Read the model definition and answer for the solid it produces. Units are mm, in the model's axes. Face numbers are marked on the shaded views. A direction names the side the tool comes from. Coordinates: 2 decimals unless noted, no trailing zeros. Write each loop counter-clockwise with the first axis right and the second up, starting at its lowest first coordinate (ties: lowest second). Pieces come first, ordered by that corner, then holes.
1) The part is cut by section D-D (y = 47.5). Determine the outline of the cut face in (x, z), then the cut area to 3 significant figures.
2) The part is cut by section C-C (y = 54). Determine the outline of the cut face in (x, z), then the cut area to 3 significant figures.
3) The part is cut by section B-B (x = 0). Determine the outline of the cut face in (y, z), then the cut area to 3 significant figures.
4) Each of these flat-tipped pins is pushed along its axis until it touches: pin 1 Ø4 at (y, z) = (27, -20) entering from +X; pin 2 Ø6 at (x, z) = (10, 12.5) entering from -Y; pin 3 Ø12 at (y, z) = (36.5, -21.5) entering from -X. Where does it stop, or does it pass through?
5) The part is cut by section A-A (z = 0). Determine the outline of the cut face in (x, y), then the cut area to 3 significant figures.
6) Which of the six approach directions +Z, -Z, +X, -X, +Y, -Y give full straight-line access (tool end or side, diameter ignored) to the marked faces 1 and 2?
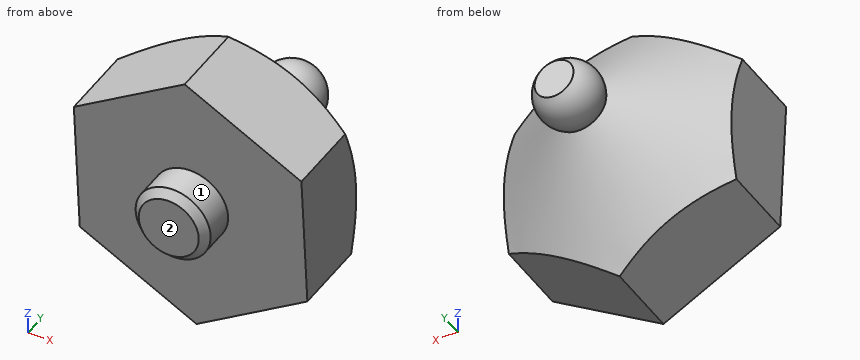
from build123d import *

# Parameters (mm, degrees)
SKETCH2_OUTSIDE_W  = 95.562
SKETCH2_OUTSIDE_H  = 95.562
CUT_EXTRUDE1_DEPTH = 80.973294862
CHAMFER1_SIZE      = 2


with BuildPart() as part:
    # Sketch1 → Revolve1 (revolve)
    with BuildSketch(Plane.XY):
        with BuildLine():
            Line((-7.160370484, 51.149500409), (-35.047619048, 30))
            Line((-35.047619048, 30), (-35.047619048, 10))
            Line((-35.047619048, 10), (-10, 10))
            Line((-10, 10), (-10, 0))
            Line((-10, 0), (0, 0))
            Line((0, 0), (0, 62.761904762))
            Line((0, 62.761904762), (-5.182953714, 62.761904762))
            ThreePointArc((-5.182953714, 62.761904762), (-8.473570486, 57.347682757), (-7.160370484, 51.149500409))
        make_face()
    revolve(axis=Axis((0, 62.761904762, 0), (0, -1, 0)))

    # Sketch2 outside → Cut-Extrude1 (cut, through all)
    with BuildSketch(Plane(origin=(0, 62.761904762, 0), x_dir=(1, 0, 0), z_dir=(0, 1, 0))):
        Rectangle(SKETCH2_OUTSIDE_W, SKETCH2_OUTSIDE_H)
        Polygon((-31.112953649, -16.134426428), (-1.583653662, -35.011821461), (29.529299986, -18.877395033), (31.112953649, 16.134426428), (1.583653662, 35.011821461), (-29.529299986, 18.877395033), align=None, mode=Mode.SUBTRACT)
    extrude(amount=-CUT_EXTRUDE1_DEPTH, mode=Mode.SUBTRACT)

    # Chamfer1
    chamfer1_edges = [part.edges().sort_by_distance(p)[0] for p in [
        (10, 0, 0),
    ]]
    chamfer(chamfer1_edges, length=CHAMFER1_SIZE)


solid = part.part
Reported:
1. outline: circle Ø23.95 at (0, 0)
1. area: 450 mm2
2. outline: circle Ø16.76 at (0, 0)
2. area: 221 mm2
3. outline: (0, -8) - (2, -10) - (10, -10) - (10, -34.19) - (30.65, -34.19) - (51.15, -7.16) arc R8.6 ccw to (62.76, -5.18) - (62.76, 5.18) arc R8.6 ccw to (51.15, 7.16) - (30.65, 34.19) - (10, 34.19) - (10, 10) - (2, 10) - (0, 8) - close
3. area: 2,640 mm2
4. pin 1: stops at x = 28.19
4. pin 2: stops at y = 10
4. pin 3: stops at x = -27.8
5. outline: (-30.38, 10) - (-10, 10) - (-10, 2) - (-8, 0) - (8, 0) - (10, 2) - (10, 10) - (30.38, 10) - (30.38, 33.54) - (7.16, 51.15) arc R8.6 ccw to (5.18, 62.76) - (-5.18, 62.76) arc R8.6 ccw to (-7.16, 51.15) - (-30.38, 33.54) - close
5. area: 2,470 mm2
6. face 1: -Y
6. face 2: +Z, -Z, +X, -X, -Y
